For this review, take the finished solid that the model builds, in its own axes (mm). Round coordinates to 2 decimals unless told otherwise and drop trailing zeros. Order: outer loops, then holes, each group sorted by start corner. A loop starts at its lowest first (then second) coordinate and runs counter-clockwise, first axis right, second up. Notation, with made-up numbers: M -27,-14 L -9,-14 A20 cw -9,-4 Z; hole C 54.25,10 d1. An arc over 180 degrees is marked long. Use a Markdown table: item, result.
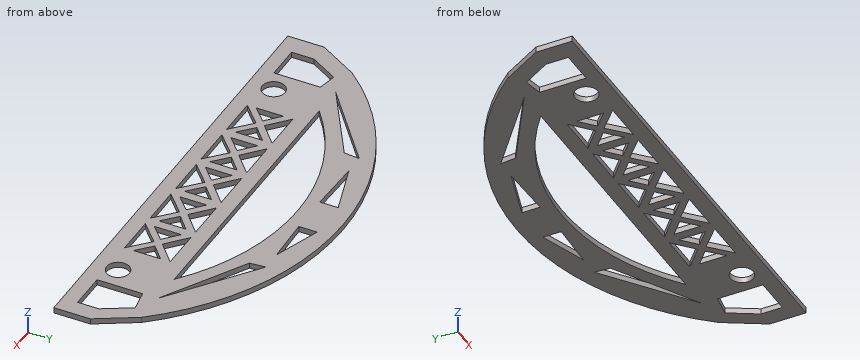
from build123d import *

# Parameters (mm, degrees)
F0_R     = 5
F1_DEPTH = 2.5


with BuildPart() as f1:
    # F0 (on Top) → F1 (new body)
    with BuildSketch(Plane.XY):
        with BuildLine():
            Line((-97.14, -17.320508), (-97.14, -33.320508))
            Line((-97.14, -33.320508), (-63.639122, -33.320508))
            Line((-63.639122, -33.320508), (69.360878, -33.320508))
            Line((69.360878, -33.320508), (102.861755, -33.320508))
            Line((102.861755, -33.320508), (102.861755, -17.320001))
            Line((102.861755, -17.320001), (92.860878, 0))
            ThreePointArc((92.860878, 0), (2.860439, 42.320725), (-87.14, 0))
            Line((-87.14, 0), (-97.14, -17.320508))
        make_face()
        Polygon((-88.377581, -17.320508), (-81.28519, -5.036127), (-73.14, -6.674613), (-73.14, -27.124608), (-88.377581, -27.124608), align=None, mode=Mode.SUBTRACT)
        with Locations((-63.639122, -22.320508)):
            Circle(F0_R, mode=Mode.SUBTRACT)
        Polygon((-31.839122, -26.674613), (-49.639122, -26.674613), (-40.739122, -18.327324), align=None, mode=Mode.SUBTRACT)
        Polygon((-49.639122, -10.879502), (-43.163221, -16.674613), (-49.639122, -22.748346), align=None, mode=Mode.SUBTRACT)
        Polygon((-31.839122, -22.748346), (-38.315108, -16.674533), (-31.839122, -10.879346), align=None, mode=Mode.SUBTRACT)
        Polygon((-27.839122, -10.879502), (-21.363221, -16.674613), (-27.839122, -22.748346), align=None, mode=Mode.SUBTRACT)
        Polygon((-10.039122, -26.674613), (-27.839122, -26.674613), (-18.939122, -18.327324), align=None, mode=Mode.SUBTRACT)
        Polygon((11.760878, -26.674613), (-6.039122, -26.674613), (2.860878, -18.327324), align=None, mode=Mode.SUBTRACT)
        Polygon((-10.039122, -22.748346), (-16.515108, -16.674533), (-10.039122, -10.879346), align=None, mode=Mode.SUBTRACT)
        Polygon((-6.039122, -10.879502), (0.436779, -16.674613), (-6.039122, -22.748346), align=None, mode=Mode.SUBTRACT)
        Polygon((-40.739122, -14.638986), (-49.639122, -6.674613), (-31.839122, -6.674613), align=None, mode=Mode.SUBTRACT)
        Polygon((-27.839122, -6.674613), (-10.039122, -6.674613), (-18.939122, -14.638986), align=None, mode=Mode.SUBTRACT)
        Polygon((33.560878, -26.674613), (15.760878, -26.674613), (24.660878, -18.327324), align=None, mode=Mode.SUBTRACT)
        Polygon((11.760878, -22.748346), (5.284892, -16.674533), (11.760878, -10.879346), align=None, mode=Mode.SUBTRACT)
        Polygon((15.760878, -10.879502), (22.236779, -16.674613), (15.760878, -22.748346), align=None, mode=Mode.SUBTRACT)
        Polygon((55.360878, -26.674613), (37.560878, -26.674613), (46.460878, -18.327324), align=None, mode=Mode.SUBTRACT)
        Polygon((33.560878, -22.748346), (27.084892, -16.674533), (33.560878, -10.879346), align=None, mode=Mode.SUBTRACT)
        Polygon((37.560878, -10.879502), (44.036779, -16.674613), (37.560878, -22.748346), align=None, mode=Mode.SUBTRACT)
        Polygon((55.360878, -22.748346), (48.884892, -16.674533), (55.360878, -10.879346), align=None, mode=Mode.SUBTRACT)
        with Locations((69.360878, -22.320508)):
            Circle(F0_R, mode=Mode.SUBTRACT)
        Polygon((88.384643, -5.036127), (95.477571, -17.320001), (95.477571, -26.674613), (78.860878, -26.674613), (78.860878, -6.674613), align=None, mode=Mode.SUBTRACT)
        Polygon((-6.039122, -6.674613), (11.760878, -6.674613), (2.860878, -14.638986), align=None, mode=Mode.SUBTRACT)
        Polygon((15.760878, -6.674613), (33.560878, -6.674613), (24.660878, -14.638986), align=None, mode=Mode.SUBTRACT)
        Polygon((37.560878, -6.674613), (55.360878, -6.674613), (46.460878, -14.638986), align=None, mode=Mode.SUBTRACT)
        Polygon((-38.47, 28.201407), (-39.14, 21.242104), (-73.14, 0), align=None, mode=Mode.SUBTRACT)
        with BuildLine():
            ThreePointArc((-59.14, 0), (2.860439, 22.360707), (64.860878, 0))
            Line((64.860878, 0), (0, 0))
            Line((0, 0), (-59.14, 0))
        make_face(mode=Mode.SUBTRACT)
        Polygon((-29.57, 28.201407), (-6.139122, 35.526987), (-6.139122, 27.468849), align=None, mode=Mode.SUBTRACT)
        Polygon((78.860878, 0), (42.000439, 21.242104), (41.330439, 28.201407), align=None, mode=Mode.SUBTRACT)
        Polygon((11.860878, 27.468849), (11.860878, 35.526987), (32.430439, 28.201407), align=None, mode=Mode.SUBTRACT)
    extrude(amount=F1_DEPTH)


solid = f1.part
Q1. Add section B-B (y = 33). Write out the cut boundary in (x, z), then the cut area to 3 significant figures.
Determined:
| item | result |
|---|---|
| outline | M -42.87,0 L -14.22,0 L -14.22,2.5 L -42.87,2.5 Z; M -6.14,0 L 11.86,0 L 11.86,2.5 L -6.14,2.5 Z; M 18.96,0 L 48.59,0 L 48.59,2.5 L 18.96,2.5 Z |
| area | 191 mm^2 |
Q2. Wall thickness on line 1 along X through (y, z) = (10.5, 1.3); line 2 along Y through (x, z) = (6.5, 1.5); line 3 along Y through (x, z) = (32.5, 1.5): over which ranges is each line inside the solid? List them lowest first. Write a range as [from, to].
Determined:
| item | result |
|---|---|
| line 1 | x = [-77.29, -60.23], [-56.33, -43.65], [49.37, 60.64], [64.89, 83.01] |
| line 2 | y = [-33.32, -26.67], [-21.74, -17.81], [-15.59, -11.38], [-6.67, 0], [22.29, 42.26] |
| line 3 | y = [-33.32, -26.67], [-25.68, -21.75], [-11.83, -7.62], [-6.67, 0], [17.73, 38.5] |
Q3. Add section D-D (z = 1.55). Give the number of separate pieces and of enclosed holes in the cut face, then the cut area to 3 significant figures.
Determined:
| item | result |
|---|---|
| separate pieces | 1 |
| enclosed holes | 29 |
| area | 7,620 mm^2 |
Q4. Add section C-C (x = -56.5). Write out the cut boundary in (y, z).
Determined:
| item | result |
|---|---|
| outline | M -33.32,0 L 0,0 L 0,2.5 L -33.32,2.5 Z; M 2.11,0 L 10.4,0 L 10.4,2.5 L 2.11,2.5 Z; M 13.54,0 L 26.12,0 L 26.12,2.5 L 13.54,2.5 Z |
Q5. Add section A-A (y = 6.5). Write out the cut boundary in (x, z).
Determined:
| item | result |
|---|---|
| outline | M -81.33,0 L -65.15,0 L -65.15,2.5 L -81.33,2.5 Z; M -62.74,0 L -50.33,0 L -50.33,2.5 L -62.74,2.5 Z; M 56.06,0 L 67.58,0 L 67.58,2.5 L 56.06,2.5 Z; M 70.21,0 L 87.06,0 L 87.06,2.5 L 70.21,2.5 Z |
Q6. Clearance check with flat-ended pins moving along their axes: pin 1 (16 mm diameter, centred on x = 69.36, y = -22.32, fed in from +Z); pin 2 (0.8 mm diameter, centred on x = -80.5, z = 1.5, fed in from +Y); pin 3 (1.2 mm diameter, centred on x = -22.5, z = 2, fed in from +Y); pin 4 (1.2 mm diameter, centred on x = 26.5, z = 1, fed in from +Y). State where each tip first meets the part, or that it passes through.
Determined:
| item | result |
|---|---|
| pin 1 | stops at z = 2.5 |
| pin 2 | stops at y = 7.76 |
| pin 3 | stops at y = 39.67 |
| pin 4 | stops at y = 40.03 |
